Here's how the part is built. I have some questions about the finished solid (model axes, mm). A direction names the side the tool comes from. Give positions to 0.01 mm unless a question says otherwise; leave off trailing zeros. Loops run counter-clockwise (first coordinate to the right, second up) from the corner with the lowest first, then second, coordinate; pieces in that order, holes last. Notation, with made-up numbers: (-33.75, 89) - (13.25, 89) arc R22 ccw to (13.25, 122) - close; hole circle Ø5 at (-29, 19). An arc over 180 degrees is marked (long way). One line per item, written item: value. Start each with the question number.
```python
from build123d import *

# Parameters (mm, degrees)
F0_W     = 40
F0_H     = 16.429857
F0_R     = 14.425633
F1_DEPTH = 25


with BuildPart() as f1:
    # F0 (on Front) → F1 (new body)
    with BuildSketch(Plane.XZ):
        with BuildLine():
            Line((-2.529519, 54.480218), (-52.529519, 54.480218))
            Line((-52.529519, 54.480218), (-52.529519, -42.776029))
            Line((-52.529519, -42.776029), (-2.529519, -42.776029))
            Line((-2.529519, -42.776029), (-2.529519, -62.283013))
            Line((-2.529519, -62.283013), (117.470481, -62.283013))
            Line((117.470481, -62.283013), (117.470481, -52.776029))
            ThreePointArc((117.470481, -52.776029), (120.399413, -45.704961), (127.470481, -42.776029))
            Line((127.470481, -42.776029), (167.470481, -42.776029))
            Line((167.470481, -42.776029), (167.470481, 54.480218))
            Line((167.470481, 54.480218), (127.470481, 54.480218))
            ThreePointArc((127.470481, 54.480218), (120.399413, 57.40915), (117.470481, 64.480218))
            Line((117.470481, 64.480218), (117.470481, 74.800561))
            Line((117.470481, 74.800561), (-2.529519, 74.800561))
            Line((-2.529519, 74.800561), (-2.529519, 54.480218))
        make_face()
        with BuildLine():
            Line((-7.529519, -32.718264), (-42.529519, -32.718264))
            Line((-42.529519, -32.718264), (-42.529519, -12.32258))
            Line((-42.529519, -12.32258), (-2.529519, -12.32258))
            Line((-2.529519, -12.32258), (-2.529519, -27.718264))
            ThreePointArc((-2.529519, -27.718264), (-3.993985, -31.253797), (-7.529519, -32.718264))
        make_face(mode=Mode.SUBTRACT)
        with Locations((-22.529519, 5.806916)):
            Rectangle(F0_W, F0_H, mode=Mode.SUBTRACT)
        with BuildLine():
            Line((87.435027, -42.776029), (22.504957, -42.776029))
            ThreePointArc((22.504957, -42.776029), (15.433889, -39.847097), (12.504957, -32.776029))
            Line((12.504957, -32.776029), (12.504957, 12.669074))
            Line((12.504957, 12.669074), (52.470481, 12.669074))
            Line((52.470481, 12.669074), (97.435027, 12.669074))
            Line((97.435027, 12.669074), (97.435027, -32.776029))
            ThreePointArc((97.435027, -32.776029), (94.506095, -39.847097), (87.435027, -42.776029))
        make_face(mode=Mode.SUBTRACT)
        with Locations((141.896114, -22.304697)):
            Circle(F0_R, mode=Mode.SUBTRACT)
        with BuildLine():
            ThreePointArc((-7.529519, 44.332098), (-3.993985, 42.867632), (-2.529519, 39.332098))
            Line((-2.529519, 39.332098), (-2.529519, 23.936415))
            Line((-2.529519, 23.936415), (-42.529519, 23.936415))
            Line((-42.529519, 23.936415), (-42.529519, 44.332098))
            Line((-42.529519, 44.332098), (-7.529519, 44.332098))
        make_face(mode=Mode.SUBTRACT)
        with BuildLine():
            ThreePointArc((12.504957, 44.480218), (15.433889, 51.551286), (22.504957, 54.480218))
            Line((22.504957, 54.480218), (87.435027, 54.480218))
            ThreePointArc((87.435027, 54.480218), (94.506095, 51.551286), (97.435027, 44.480218))
            Line((97.435027, 44.480218), (97.435027, 34.150277))
            Line((97.435027, 34.150277), (12.504957, 34.150277))
            Line((12.504957, 34.150277), (12.504957, 44.480218))
        make_face(mode=Mode.SUBTRACT)
        with Locations((141.896114, 34.150277)):
            Circle(F0_R, mode=Mode.SUBTRACT)
    extrude(amount=F1_DEPTH)


solid = f1.part
```
(1) Will these pins go through, and if not, where does the flat tip stop? pin 1 (7.5 mm diameter, centred on x = -16.5, y = -7.5, fed in from -Z); pin 2 (1.5 mm diameter, centred on x = 119.5, y = -11.5, fed in from -Z); pin 3 (7.5 mm diameter, centred on x = 153.5, y = -12, fed in from +Z).
(2) Please list where these lines run through material, in increasing order: probe 1 along X at (y, z) = (-1.25, 4); probe 2 along Z at (x, y) = (-24.5, -8.75); probe 3 along Z at (x, y) = (53.5, -6.5). Write a range as from..to.
(3) If we section it at C-C on y = -11.75: Give the number of separate pieces and of enclosed holes in the cut face, plus the area to 3 significant figures.
(4) If we section it at A-A on z = 7: List the corners of the cut face in (x, y) for me.
(5) If we section it at B-B on x = 83: List the corners of the cut face in (y, z) for me, plus the area to 3 significant figures.
(6) For faces 1 (the face through (58, -12, 74.801)), 2 (the face through (56, -25, 22)), 3 (the face through (148, -12, 54.48)), 4 (the face through (-28, -12, -42.776)), 5 (the face through (94.428, -12.325, 51.629)), which set-ups out of +Z, -Z, +X, -X, +Y, -Y let a thin tool reach every point of the face, with its end or its side?
(7) If we mould it in two halves opening along X, with no side actions, what happens to faces 6 (the face through (-2.53, -12, 32)), 7 (the face through (147, -12, -42.776)), 8 (the face through (55, -12, -42.776))? For each: pulls with the +X half, pulls with the -X half, needs draft (parallel to the pull), parting line crosses it, or undercut.
Found:
1. pin 1: z = -42.78
1. pin 2: z = -47.88
1. pin 3: z = 54.48
2. probe 1: -52.53..-42.53, -2.53..12.5, 97.44..167.47
2. probe 2: -42.78..-32.72, -12.32..-2.41, 14.02..23.94, 44.33..54.48
2. probe 3: -62.28..-42.78, 12.67..34.15, 54.48..74.8
3. separate pieces: 1
3. enclosed holes: 7
3. area: 16,300 mm^2
4. outline: (-52.53, -25) - (-42.53, -25) - (-42.53, 0) - (-52.53, 0) - close; (-2.53, -25) - (12.5, -25) - (12.5, 0) - (-2.53, 0) - close; (97.44, -25) - (167.47, -25) - (167.47, 0) - (97.44, 0) - close
5. outline: (-25, -62.28) - (0, -62.28) - (0, -42.78) - (-25, -42.78) - close; (-25, 12.67) - (0, 12.67) - (0, 34.15) - (-25, 34.15) - close; (-25, 54.48) - (0, 54.48) - (0, 74.8) - (-25, 74.8) - close
5. area: 1,530 mm^2
6. face 1: +Z, +X, -X, +Y, -Y
6. face 2: +Z, -Z, +X, -X, -Y
6. face 3: +Z, +X, +Y, -Y
6. face 4: -Z, -X, +Y, -Y
6. face 5: +Y, -Y
7. face 6: undercut
7. face 7: needs draft
7. face 8: undercut
